```python
from build123d import *

# Parameters (mm, degrees)
BOSS_EXTRUDE1_DEPTH = 8
BOSS_EXTRUDE2_DEPTH = 15
SKETCH4_R           = 5
CUT_EXTRUDE1_DEPTH  = 40
SKETCH5_R           = 5
CUT_EXTRUDE2_DEPTH  = 40
SKETCH6_R           = 5
CUT_EXTRUDE3_DEPTH  = 40


with BuildPart() as part:
    # Sketch2 → Boss-Extrude1 (new body)
    with BuildSketch(Plane(origin=(0, 0, 0), x_dir=(1, 0, 0), z_dir=(0, 1, 0))):
        Polygon((-62.5, -54.126587737), (62.5, -54.126587737), (0, 54.126587737), align=None)
    extrude(amount=BOSS_EXTRUDE1_DEPTH)

    # Sketch3 → Boss-Extrude2 (add)
    with BuildSketch(Plane(origin=(0, 8, 0), x_dir=(1, 0, 0), z_dir=(0, 1, 0))):
        Polygon((31.25, 0), (18.75, 21.650635095), (5.759618943, 14.150635095), (30.759618943, -29.150635095), (43.75, -21.650635095), align=None)
        Polygon((0, -54.126587737), (25, -54.126587737), (25, -39.126587737), (-25, -39.126587737), (-25, -54.126587737), align=None)
        Polygon((-31.25, 0), (-43.75, -21.650635095), (-30.759618943, -29.150635095), (-5.759618943, 14.150635095), (-18.75, 21.650635095), align=None)
    extrude(amount=BOSS_EXTRUDE2_DEPTH)

    # Sketch4 → Cut-Extrude1 (cut)
    with BuildSketch(Plane(origin=(25, 0, 0), x_dir=(0, 0, -1), z_dir=(1, 0, 0))):
        with Locations((-46.626587737, 15.5)):
            Circle(SKETCH4_R)
    extrude(amount=-CUT_EXTRUDE1_DEPTH, mode=Mode.SUBTRACT)

    # Sketch5 → Cut-Extrude2 (cut)
    with BuildSketch(Plane(origin=(20.3125, 0, 35.182282029), x_dir=(0.866025404, 0, -0.5), z_dir=(0.5, 0, 0.866025404))):
        with Locations((19.563293868, 15.5)):
            Circle(SKETCH5_R)
    extrude(amount=-CUT_EXTRUDE2_DEPTH, mode=Mode.SUBTRACT)

    # Sketch6 → Cut-Extrude3 (cut)
    with BuildSketch(Plane(origin=(4.6875, 0, -8.11898816), x_dir=(-0.866025404, 0, -0.5), z_dir=(0.5, 0, -0.866025404))):
        with Locations((19.563293868, 15.5)):
            Circle(SKETCH6_R)
    extrude(amount=-CUT_EXTRUDE3_DEPTH, mode=Mode.SUBTRACT)


solid = part.part
```
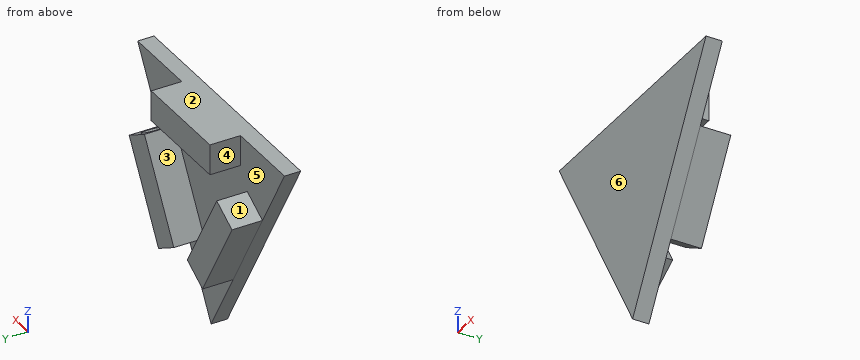
Read the model definition and answer for the solid it produces. Units are mm, in the model's axes. Face numbers are marked on the shaded views. A direction names the side the tool comes from. Coordinates: 2 decimals unless noted, no trailing zeros. Loops run counter-clockwise (first coordinate to the right, second up) from the corner with the lowest first, then second, coordinate; pieces in that order, holes last. Notation, with made-up numbers: (73.5, -25.5) - (101.5, -25.5) arc R32 cw to (101.5, 1.5) - close; hole circle Ø11 at (34, 51.25). An arc over 180 degrees is marked (long way). Answer in a Markdown table with one row per item.
1. Straight lines are drawn through the part: line 1 (X direction, y = 12.25, z = 6.5); line 2 (X direction, y = 16.5, z = -6); line 3 (Y direction, x = 24.5, z = 27). For each, find the intervals that lie inside material, in ascending order.
Conclusion:
| item | result |
|---|---|
| line 1 | x = -35 to -30.73, -21.96 to -17.68, 17.68 to 21.96, 30.73 to 35 |
| line 2 | x = -27.79 to -24.78, -13.47 to -10.47, 10.47 to 13.47, 24.78 to 27.79 |
| line 3 | y = 0 to 8 |
2. Find section A-A, the plane y = 18.5. Write down the section's boundary in (x, z), then the cut area to 3 significant figures.
Conclusion:
| item | result |
|---|---|
| outline | (-43.75, 21.65) - (-18.75, -21.65) - (-15.72, -19.9) - (-35.72, 14.74) - (-28.79, 18.74) - (-8.79, -15.9) - (-5.76, -14.15) - (-30.76, 29.15) - close; (-25, 39.13) - (25, 39.13) - (25, 42.63) - (-15, 42.63) - (-15, 50.63) - (25, 50.63) - (25, 54.13) - (-25, 54.13) - close; (5.76, -14.15) - (18.75, -21.65) - (43.75, 21.65) - (40.72, 23.4) - (20.72, -11.24) - (13.79, -7.24) - (33.79, 27.4) - (30.76, 29.15) - close |
| area | 1,290 mm² |
3. Find section B-B, the plane z = 44. Write down the section's boundary in (x, y), then the cut area to 3 significant figures.
Conclusion:
| item | result |
|---|---|
| outline | (-56.65, 0) - (56.65, 0) - (56.65, 8) - (25, 8) - (25, 11.25) - (-15, 11.25) - (-15, 19.75) - (25, 19.75) - (25, 23) - (-25, 23) - (-25, 8) - (-56.65, 8) - close |
| area | 1,320 mm² |
4. Find section D-D, the plane z = -4.5. Count the separate pieces of the cut face and the enclosed holes in it, then the cut area to 3 significant figures.
Conclusion:
| item | result |
|---|---|
| separate pieces | 1 |
| enclosed holes | 2 |
| area | 797 mm² |
5. Determine the mould class of the marked faces 3, 4, 5 and 6 for opening direction X: +X half, -X half, draft (parallel to the pull), parting line (faces both ways), or undercut.
Conclusion:
| item | result |
|---|---|
| face 3 | undercut |
| face 4 | -X half |
| face 5 | undercut |
| face 6 | draft |
6. Find section C-C, the plane y = 4.25. Write down the section's boundary in (x, z), then the cut area to 3 significant figures.
Conclusion:
| item | result |
|---|---|
| outline | (-62.5, 54.13) - (0, -54.13) - (62.5, 54.13) - close |
| area | 6,770 mm² |
7. Which of the six approach directions +Z, -Z, +X, -X, +Y, -Y give full straight-line access (tool end or side, diameter ignored) to the marked faces 1 and 2?
Conclusion:
| item | result |
|---|---|
| face 1 | +Z, -X, +Y |
| face 2 | +Z, +X, -X, +Y, -Y |
8. Given pin 1 (8 mm diameter, centred on y = 17, z = 42.5, fed in from +X); pin 2 (5 mm diameter, centred on x = -2, y = 19.5, fed in from -Z); pin 3 (13 mm diameter, centred on y = 15.5, z = 46.63, fed in from -X), each flat-ended and moving along its own axis, determine where each tip first touches the part or whether it passes through.
Conclusion:
| item | result |
|---|---|
| pin 1 | stops at x = 25 |
| pin 2 | stops at z = 39.13 |
| pin 3 | stops at x = -25 |
